Answer from the drawing. Dimensions are ordinates in mm from the lowest x, y and z of the part. Coordinates: 2 decimals unless noted, no trailing zeros. Write each loop counter-clockwise with the first axis right and the second up, starting at its lowest first coordinate (ties: lowest second). Pieces come first, ordered by that corner, then holes. Notation, with made-up numbers: (65, 67.25) -> (98, 67.25) arc R34 cw to (98, 99.25) -> close; hole circle Ø8 at (46.5, 17). An arc over 180 degrees is marked (long way). Answer as a JSON object with one key per item and string values. Group by question number.
(1) Find section C-C (y = 0.35). Give the vertices of the cut face in (x, z).
(2) Find section B-B (z = 2.5). Give the vertices of the cut face in (x, y), then the cut area to 3 significant figures.
(3) Find section D-D (z = 7). Give the vertices of the cut face in (x, y), then the cut area to 3 significant figures.
(4) Straight lines are drawn through the part: L1, parallel to X at y = 0.55, z = 2.5; L2, parallel to Y at x = 7.5, z = 1; L3, parallel to Z at x = 7.5, y = 1.15. For each, find the intervals that lie inside material, in ascending order.
(5) Flat-ended cylindrical pins translate along their axes: P1, Ø0.5, axis at x = 8.5, y = 1.5, coming from the +Z side; P2, Ø0.5, axis at x = 9, y = 1.5, coming from the -Z side; P3, Ø1, axis at x = 4, z = 2.5, coming from the +Y side. Find the tip coordinate at first contact, or state that the pin passes through.
(6) Find section A-A (x = 15.5). Give the vertices of the cut face in (y, z).
(7) For a pull along Y with two mould halves and no side action, classify the marked faces 1 and 2 as +Y half, -Y half, draft (parallel to the pull), parting line (faces both ways), or undercut.
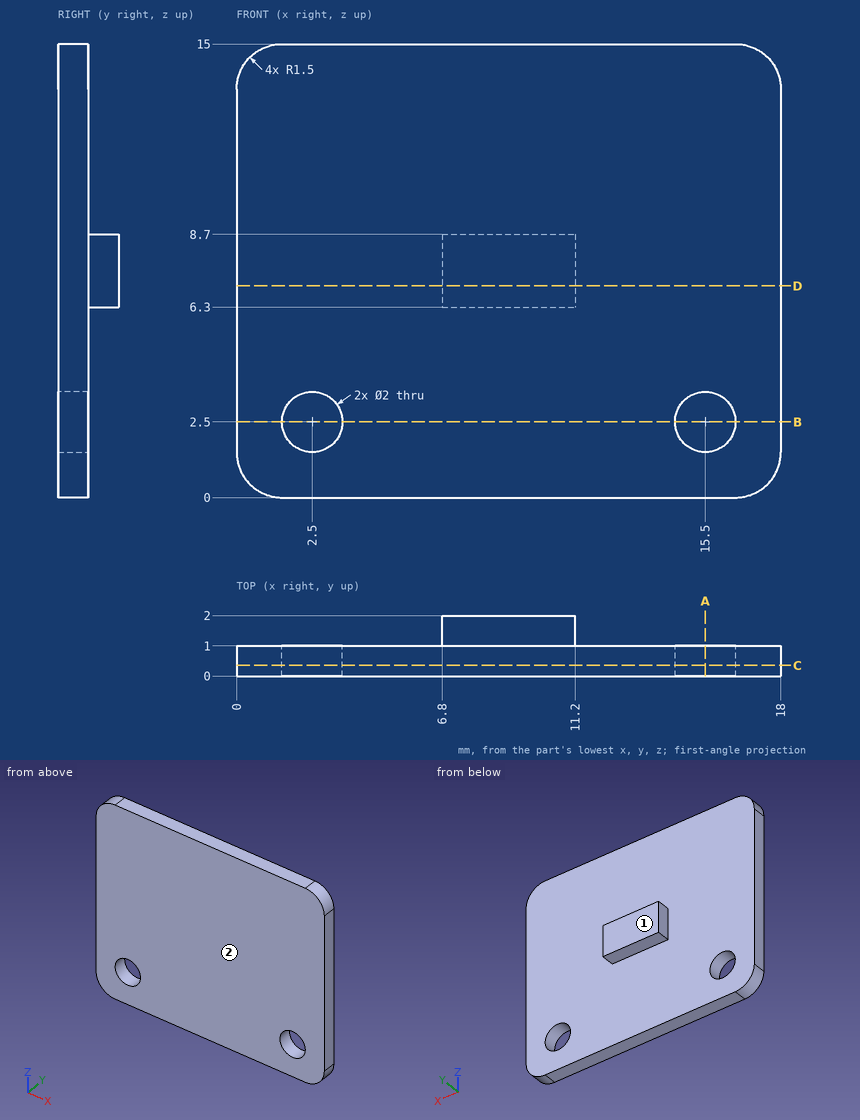
Results below:
{
 "1": {"outline": "(0, 1.5) arc R1.5 ccw to (1.5, 0) -> (16.5, 0) arc R1.5 ccw to (18, 1.5) -> (18, 13.5) arc R1.5 ccw to (16.5, 15) -> (1.5, 15) arc R1.5 ccw to (0, 13.5) -> close; hole circle Ø2 at (2.5, 2.5); hole circle Ø2 at (15.5, 2.5)"},
 "2": {"outline": "(0, 0) -> (1.5, 0) -> (1.5, 1) -> (0, 1) -> close; (3.5, 0) -> (14.5, 0) -> (14.5, 1) -> (3.5, 1) -> close; (16.5, 0) -> (18, 0) -> (18, 1) -> (16.5, 1) -> close", "area": "14.0 mm2"},
 "3": {"outline": "(0, 0) -> (18, 0) -> (18, 1) -> (11.2, 1) -> (11.2, 2) -> (6.8, 2) -> (6.8, 1) -> (0, 1) -> close", "area": "22.4 mm2"},
 "4": {"L1": "x = 0 to 1.5, 3.5 to 14.5, 16.5 to 18", "L2": "y = 0 to 1", "L3": "z = 6.3 to 8.7"},
 "5": {"P1": "stops at z = 8.7", "P2": "stops at z = 6.3", "P3": "stops at y = 1"},
 "6": {"outline": "(0, 0) -> (1, 0) -> (1, 1.5) -> (0, 1.5) -> close; (0, 3.5) -> (1, 3.5) -> (1, 15) -> (0, 15) -> close"},
 "7": {"face 1": "+Y half", "face 2": "-Y half"}
}
